from build123d import *

# Parameters (mm, degrees)
SKETCH1_W          = 3.5
SKETCH1_H          = 6.05
SKETCH1_W_2        = 15.5
SKETCH1_H_2        = 1.05
SKETCH2_R          = 1.75
CUT_EXTRUDE1_DEPTH = 23.06059836
CIRPATTERN1_COUNT  = 4


with BuildPart() as part:
    # Sketch1 → Revolve1 (revolve)
    with BuildSketch(Plane.XY, mode=Mode.PRIVATE) as revolve1_sk:
        with Locations((11.75, 8.075)):
            Rectangle(SKETCH1_W, SKETCH1_H)
        with Locations((7.75, 4.525)):
            Rectangle(SKETCH1_W_2, SKETCH1_H_2)
    revolve(revolve1_sk.sketch.rotate(Axis((0, 0, 0), (1, 0, 0)), 90), axis=Axis((0, 0, 0), (1, 0, 0)))

    # Sketch2 → Cut-Extrude1 (cut, through all)
    with BuildSketch(Plane(origin=(0, 0, 0), x_dir=(0, 0, -1), z_dir=(1, 0, 0))):
        with Locations((8, 0)):
            Circle(SKETCH2_R)
    cut_extrude1 = extrude(amount=CUT_EXTRUDE1_DEPTH, mode=Mode.SUBTRACT)

    # CirPattern1: Cut-Extrude1 ×4 about axis
    cirpattern1_axis = Axis((0, 0, 0), (1, 0, 0))
    for i in range(1, CIRPATTERN1_COUNT):
        add(cut_extrude1.rotate(cirpattern1_axis, i * 360 / CIRPATTERN1_COUNT), mode=Mode.SUBTRACT)


solid = part.part
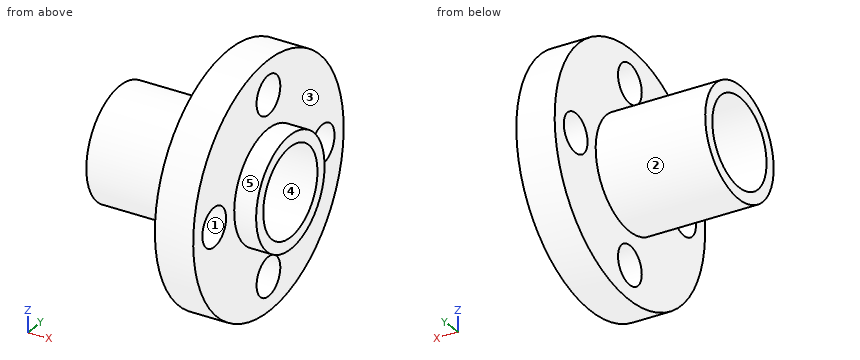
Source: CAD feature listing. Evaluate the final solid. Frame: model axes, mm. Face numbers are marked on the shaded views. A direction names the side the tool comes from. Coordinates: 2 decimals unless noted, no trailing zeros. Order: outer loops, then holes, each group sorted by start corner. A loop starts at its lowest first (then second) coordinate and runs counter-clockwise, first axis right, second up.
Item 1: Set-up query: the marked faces 1 and 2. Return all of +Z, -Z, +X, -X, +Y, -Y with unobstructed straight access to the full face (end or side cutting, diameter ignored); none if empty.
Output values:
face 1: +X, -X
face 2: -X
Item 2: First-contact query: P1, Ø1.5, axis at x = 2, z = -0.5, coming from the +Y side; P2, Ø3, axis at x = 2.5, z = 3, coming from the -Y side; P3, Ø8, axis at x = 8, y = 5, coming from the -Z side. Flat tips, straight axial feed; report the tip coordinate or a pass-through.
Output values:
P1: stops at y = 5.05
P2: stops at y = -4.82
P3: stops at z = -10.99
Item 3: Cut plane C-C (x = 13). Return loops of the section in (y, z), plus the area to 3 significant figures.
Output values:
outline: circle Ø22.2 at (0, 0); hole circle Ø3.5 at (-8, 0); hole circle Ø8 at (0, 0); hole circle Ø3.5 at (0, -8); hole circle Ø3.5 at (0, 8); hole circle Ø3.5 at (8, 0)
area: 298 mm2
Item 4: Cut plane A-A (y = 0). Return loops of the section in (x, z), plus the area to 3 significant figures.
Output values:
outline: (0, -5.05) - (10, -5.05) - (10, -6.25) - (13.5, -6.25) - (13.5, -5.05) - (15.5, -5.05) - (15.5, -4) - (0, -4) - close; (0, 4) - (15.5, 4) - (15.5, 5.05) - (13.5, 5.05) - (13.5, 6.25) - (10, 6.25) - (10, 5.05) - (0, 5.05) - close; (10, -11.1) - (13.5, -11.1) - (13.5, -9.75) - (10, -9.75) - close; (10, 9.75) - (13.5, 9.75) - (13.5, 11.1) - (10, 11.1) - close
area: 50.4 mm2
Item 5: Material intervals for line 1 (Y direction, x = 10.5, z = 1.25); line 2 (X direction, y = 5, z = -3); line 3 (Y direction, x = 2, z = 0.25), sorted ascending.
Output values:
line 1: y = -11.03 to -9.22, -6.78 to -3.8, 3.8 to 6.78, 9.22 to 11.03
line 2: x = 10 to 13.5
line 3: y = -5.04 to -3.99, 3.99 to 5.04
Item 6: Pull-direction query (Z, two-part tool) for the marked faces 3, 4 and 5; classes: pulls with the +Z half, pulls with the -Z half, needs draft (parallel to the pull), parting line crosses it, or undercut.
Output values:
face 3: needs draft
face 4: undercut
face 5: parting line crosses it
Item 7: Cut plane D-D (z = 7). Return loops of the section in (x, y).
Output values:
outline: (10, -8.61) - (13.5, -8.61) - (13.5, -1.44) - (10, -1.44) - close; (10, 1.44) - (13.5, 1.44) - (13.5, 8.61) - (10, 8.61) - close
